Source: three-view drawing plus pictorial views. Frame: mm from the lowest corner of the part. A direction names the side the tool comes from. Give positions to 0.01 mm unless a question says otherwise; leave off trailing zeros. Write each loop counter-clockwise with the first axis right and the second up, starting at its lowest first coordinate (ties: lowest second). Pieces come first, ordered by that corner, then holes.
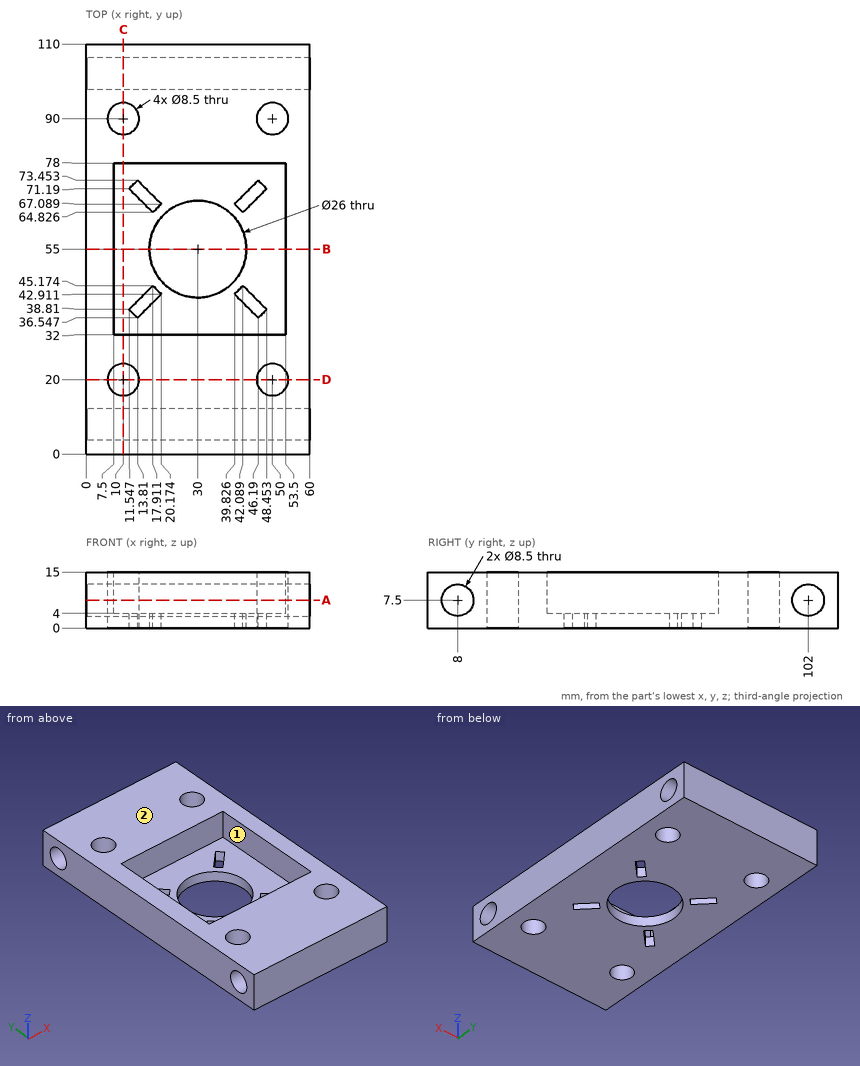
Q1. Pin query (flat end, axial travel): P1, Ø5.5, axis at x = 31, z = 9, coming from the -Y side; P2, Ø14, axis at x = 37, y = 52.5, coming from the +Z side. Return the tip coordinate at first contact, or that it passes through.
Filled sheet:
P1: stops at y = 0
P2: stops at z = 4
Q2. Section C-C on x = 10. Output: boundary loops of the cut face in (y, z).
Filled sheet:
outline: (0, 0) - (15.75, 0) - (15.75, 15) - (0, 15) - close; (24.25, 0) - (85.75, 0) - (85.75, 15) - (78, 15) - (78, 4) - (32, 4) - (32, 15) - (24.25, 15) - close; (94.25, 0) - (110, 0) - (110, 15) - (94.25, 15) - close; hole circle Ø8.5 at (8, 7.5); hole circle Ø8.5 at (102, 7.5)
Q3. Access query for the marked faces 1 and 2. Directions: +Z, -Z, +X, -X, +Y, -Y. A direction counts if a zero-diameter tool reaches every point of the face in a straight line with its end or side. Return the directions, or none.
Filled sheet:
face 1: +Z
face 2: +Z, +X, -X, +Y, -Y
Q4. Section D-D on y = 20. Output: boundary loops of the cut face in (x, z).
Filled sheet:
outline: (0, 0) - (5.75, 0) - (5.75, 15) - (0, 15) - close; (14.25, 0) - (45.75, 0) - (45.75, 15) - (14.25, 15) - close; (54.25, 0) - (60, 0) - (60, 15) - (54.25, 15) - close
Q5. Section A-A on z = 7.5. Output: boundary loops of the cut face in (x, y).
Filled sheet:
outline: (0, 0) - (60, 0) - (60, 3.75) - (0, 3.75) - close; (0, 12.25) - (60, 12.25) - (60, 97.75) - (0, 97.75) - close; (0, 106.25) - (60, 106.25) - (60, 110) - (0, 110) - close; hole circle Ø8.5 at (10, 20); hole circle Ø8.5 at (10, 90); hole (7.5, 32) - (53.5, 32) - (53.5, 78) - (7.5, 78) - close; hole circle Ø8.5 at (50, 20); hole circle Ø8.5 at (50, 90)
Q6. Ray query, line 1 along Y through (x, z) = (15, 7.5); line 2 along Y through (x, z) = (30, 1.65); line 3 along Y through (x, z) = (10, 7.5). Return the intervals inside material, ascending.
Filled sheet:
line 1: y = 0 to 3.75, 12.25 to 32, 78 to 97.75, 106.25 to 110
line 2: y = 0 to 42, 68 to 110
line 3: y = 0 to 3.75, 12.25 to 15.75, 24.25 to 32, 78 to 85.75, 94.25 to 97.75, 106.25 to 110
Q7. Section B-B on y = 55. Output: boundary loops of the cut face in (x, z), plus the area to 3 significant figures.
Filled sheet:
outline: (0, 0) - (17, 0) - (17, 4) - (7.5, 4) - (7.5, 15) - (0, 15) - close; (43, 0) - (60, 0) - (60, 15) - (53.5, 15) - (53.5, 4) - (43, 4) - close
area: 290 mm2
